Could you check a few things on this model? Use its own coordinates, in mm. Round coordinates to 2 decimals unless told otherwise and drop trailing zeros. Write each question's results on one line, items separated by ' | '. Start each with the question number.
(1) Imagine slicing it at A-A on x = -4.5. State how many separate pieces and enclosed holes the cut face has, then the cut area to 3 significant figures.
(2) Please list where these lines run through material, in increasing order: line 1 (Y direction, x = 12, z = 4.25); line 2 (X direction, y = -146.5, z = 3.5); line 3 (X direction, y = -128.5, z = 5.5). Write a range as [from, to].
(3) For P1, Ø1.9, axis at x = -4.5, z = 2.5, coming from the +Y side, with a flat end and sliding along its axis, tell me the tip position at first contact or that it passes through.
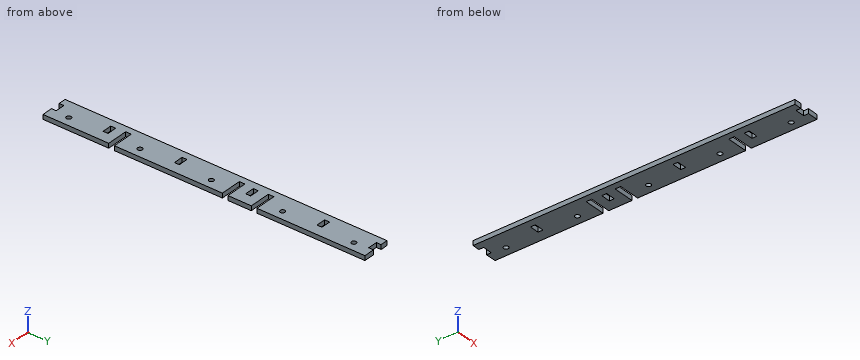
```python
from build123d import *

# Parameters (mm, degrees)
SKETCH1_W             = 38.1
SKETCH1_H             = 498.348
SKETCH1_R             = 3
BOSS_EXTRUDE1_DEPTH   = 6.35
M6_CLEARANCE_HOLE1_D  = 6.6
LPATTERN1_COUNT       = 3
LPATTERN1_PITCH       = 98.8568
LPATTERN1_COL_COUNT   = 3
LPATTERN1_COL_PITCH   = 98.8568
SKETCH4_W             = 26.9875
SKETCH4_H             = 3.175
SKETCH4_W_2           = 25.7175
CUT_EXTRUDE1_DEPTH    = 250.981813891
LPATTERN2_START       = -8.887219794
LPATTERN2_OUTLINE_W   = 6.858
LPATTERN2_OUTLINE_H   = 6.35
LPATTERN2_OUTLINE_W_2 = 6.604
LPATTERN2_DEPTH       = 13.208


# Read off the part's stored shape, not the designer's step: LPattern2
with BuildPart() as part:
    # Sketch1 → Boss-Extrude1 (new body)
    with BuildSketch(Plane.XY):
        Rectangle(SKETCH1_W, SKETCH1_H)
        with Locations((6.35, 0)):
            Circle(SKETCH1_R, mode=Mode.SUBTRACT)
    extrude(amount=BOSS_EXTRUDE1_DEPTH)

    # M6 Clearance Hole1 (through all)
    with Locations(Plane.XY.offset(6.35)):
        with Locations((6.35, 0)):
            m6_clearance_hole1 = Hole(M6_CLEARANCE_HOLE1_D / 2)

    # LPattern1: M6 Clearance Hole1 ×3
    with Locations(*[(0, -i * LPATTERN1_PITCH, 0) for i in range(1, LPATTERN1_COUNT)]):
        add(m6_clearance_hole1, mode=Mode.SUBTRACT)

    # LPattern1 col: M6 Clearance Hole1 ×3
    with Locations(*[(0, i * LPATTERN1_COL_PITCH, 0) for i in range(1, LPATTERN1_COL_COUNT)]):
        add(m6_clearance_hole1, mode=Mode.SUBTRACT)

    # Sketch4 → Cut-Extrude1 (cut, through all)
    with BuildSketch(Plane.XY.offset(6.35)):
        Polygon((-8.9535, -231.0064), (-8.9535, -223.2594), (-19.05, -223.2594), (-19.05, -249.174), (19.05, -249.174), (19.05, -231.0064), align=None)
        Polygon((19.05, -225.5454), (19.05, -223.2594), (-8.9535, -223.2594), (-8.9535, -231.0064), (19.05, -231.0064), (19.05, -228.7204), (-6.6675, -228.7204), (-6.6675, -225.5454), align=None)
        with Locations((5.55625, -128.2159)):
            Rectangle(SKETCH4_W, SKETCH4_H)
        Polygon((-10.2235, -132.0894), (19.05, -132.0894), (19.05, -129.8034), (-7.9375, -129.8034), (-7.9375, -126.6284), (19.05, -126.6284), (19.05, -124.3424), (-10.2235, -124.3424), align=None)
        with Locations((6.19125, -227.1329)):
            Rectangle(SKETCH4_W_2, SKETCH4_H)
        with Locations((5.55625, 29.3591)):
            Rectangle(SKETCH4_W, SKETCH4_H)
        Polygon((-10.2235, 25.4856), (19.05, 25.4856), (19.05, 27.7716), (-7.9375, 27.7716), (-7.9375, 30.9466), (19.05, 30.9466), (19.05, 33.2326), (-10.2235, 33.2326), align=None)
        Polygon((19.05, 71.0852), (19.05, 73.3712), (-10.2235, 73.3712), (-10.2235, 65.6242), (19.05, 65.6242), (19.05, 67.9102), (-7.9375, 67.9102), (-7.9375, 71.0852), align=None)
        with Locations((5.55625, 69.4977)):
            Rectangle(SKETCH4_W, SKETCH4_H)
        Polygon((-19.05, 249.174), (-19.05, 223.1992), (-10.2235, 223.1992), (-10.2235, 230.9462), (19.05, 230.9462), (19.05, 249.174), align=None)
        with Locations((5.55625, 227.0727)):
            Rectangle(SKETCH4_W, SKETCH4_H)
        Polygon((-10.2235, 230.9462), (-10.2235, 223.1992), (19.05, 223.1992), (19.05, 225.4852), (-7.9375, 225.4852), (-7.9375, 228.6602), (19.05, 228.6602), (19.05, 230.9462), align=None)
    extrude(amount=-CUT_EXTRUDE1_DEPTH, mode=Mode.SUBTRACT)

    # LPattern2 outline → LPattern2 (cut)
    with BuildSketch(Plane.YZ.offset(LPATTERN2_START)):
        with Locations((148.2852, 3.175)):
            Rectangle(LPATTERN2_OUTLINE_W, LPATTERN2_OUTLINE_H)
        with Locations((219.8972, 3.175)):
            Rectangle(LPATTERN2_OUTLINE_W_2, LPATTERN2_OUTLINE_H)
        with Locations((49.4284, 3.175)):
            Rectangle(LPATTERN2_OUTLINE_W, LPATTERN2_OUTLINE_H)
        with Locations((-49.4284, 3.175)):
            Rectangle(LPATTERN2_OUTLINE_W, LPATTERN2_OUTLINE_H)
        with Locations((-148.2852, 3.175)):
            Rectangle(LPATTERN2_OUTLINE_W, LPATTERN2_OUTLINE_H)
        with Locations((-219.9574, 3.175)):
            Rectangle(LPATTERN2_OUTLINE_W_2, LPATTERN2_OUTLINE_H)
    extrude(amount=LPATTERN2_DEPTH, mode=Mode.SUBTRACT)


solid = part.part
```
Response:
1) separate pieces: 8 | enclosed holes: 0 | area: 2,430 mm²
2) line 1: [-223.26, -132.09], [-124.34, 25.49], [33.23, 65.62], [73.37, 223.2] | line 2: [-19.05, -8.89], [4.32, 19.05] | line 3: [-19.05, -10.22]
3) P1: y = 216.6
